from build123d import *

# Parameters (mm, degrees)
SKETCH1_W           = 76.2
SKETCH1_H           = 127
BOSS_EXTRUDE1_DEPTH = 2.54
SKETCH2_W           = 2.54
SKETCH2_H           = 25.4
CUT_EXTRUDE1_DEPTH  = 3.54
SKETCH4_W           = 2.54
SKETCH4_H           = 25.4
CUT_EXTRUDE3_DEPTH  = 3.54
SKETCH3_W           = 2.54
SKETCH3_H           = 25.4
CUT_EXTRUDE4_DEPTH  = 3.54


with BuildPart() as part:
    # Sketch1 → Boss-Extrude1 (new body)
    with BuildSketch(Plane.XY):
        with Locations((38.1, 63.5)):
            Rectangle(SKETCH1_W, SKETCH1_H)
    extrude(amount=BOSS_EXTRUDE1_DEPTH)

    # Sketch2 → Cut-Extrude1 (cut, through all)
    with BuildSketch(Plane.XY.offset(2.54)):
        with Locations((1.27, 114.3)):
            Rectangle(SKETCH2_W, SKETCH2_H)
    extrude(amount=-CUT_EXTRUDE1_DEPTH, mode=Mode.SUBTRACT)

    # Sketch4 → Cut-Extrude3 (cut, through all)
    with BuildSketch(Plane.XY.offset(2.54)):
        with Locations((1.27, 12.7)):
            Rectangle(SKETCH4_W, SKETCH4_H)
        with Locations((74.93, 12.7)):
            Rectangle(SKETCH4_W, SKETCH4_H)
        with Locations((1.27, 63.5)):
            Rectangle(SKETCH4_W, SKETCH4_H)
        with Locations((74.93, 63.5)):
            Rectangle(SKETCH4_W, SKETCH4_H)
    extrude(amount=-CUT_EXTRUDE3_DEPTH, mode=Mode.SUBTRACT)

    # Sketch3 → Cut-Extrude4 (cut, through all)
    with BuildSketch(Plane.XY.offset(2.54)):
        with Locations((74.93, 114.3)):
            Rectangle(SKETCH3_W, SKETCH3_H)
    extrude(amount=-CUT_EXTRUDE4_DEPTH, mode=Mode.SUBTRACT)


solid = part.part
Design review of the part built by this model. Coordinates are the model's own, in mm. A direction names the side the tool comes from. Coordinates: 2 decimals unless noted, no trailing zeros. Order: outer loops, then holes, each group sorted by start corner. A loop starts at its lowest first (then second) coordinate and runs counter-clockwise, first axis right, second up. Notation, with made-up numbers: (61, 60) -> (100, 60) arc R15 cw to (100, 66) -> close; hole circle Ø3 at (25.25, 55). An arc over 180 degrees is marked (long way). Use one line per item in the form item = value. Start each with the question number.
(1) Add section B-B on y = 10. State the section outline as (x, z) points, plus the area to 3 significant figures.
(2) For probe 1 along X at (y, z) = (7, 1.45), list the stretches that pass through material, from the lowest coordinate up.
(3) The part is to be moulded in two halves that separate along Y. For faces 1 (the flat face through (73.66, 63, 1)), 2 (the flat face through (2.54, 13, 1)), 3 (the flat face through (1, 25.4, 1)), say which applies: +Y half, -Y half, draft (parallel to the pull), parting line (faces both ways), or undercut.
(4) Insertion check: pin 1 (1.3 mm diameter, centred on y = 110, z = 1.5, fed in from -X); pin 2 (0.8 mm diameter, centred on x = 75, z = 1, fed in from -Y); pin 3 (0.8 mm diameter, centred on y = 118.5, z = 2, fed in from +X). Each pin has a flat end and moves straight along its axis. Give the tip position at first contact, or say it passes through.
(5) For faces 4 (the flat face through (2.54, 114, 1)), 5 (the flat face through (75, 25.4, 1)), 6 (the flat face through (73.66, 114, 1)), list the 3-axis set-ups (+Z, -Z, +X, -X, +Y, -Y) from which the entire face can be reached by the end or side of a thin tool; tool diameter is ignored.
(6) Add section A-A on z = 0.9. State the section outline as (x, y) points.
Answer block:
q1.outline = (2.54, 0) -> (73.66, 0) -> (73.66, 2.54) -> (2.54, 2.54) -> close
q1.area = 181 mm²
q2.probe_1 = 2.54 to 73.66
q3.face_1 = undercut
q3.face_2 = draft
q3.face_3 = -Y half
q4.pin_1 = 2.54
q4.pin_2 = 25.4
q4.pin_3 = 73.66
q5.face_4 = +Z, -Z, -X, +Y
q5.face_5 = +Z, -Z, +X, -Y
q5.face_6 = +Z, -Z, +X, +Y
q6.outline = (0, 25.4) -> (2.54, 25.4) -> (2.54, 0) -> (73.66, 0) -> (73.66, 25.4) -> (76.2, 25.4) -> (76.2, 50.8) -> (73.66, 50.8) -> (73.66, 76.2) -> (76.2, 76.2) -> (76.2, 101.6) -> (73.66, 101.6) -> (73.66, 127) -> (2.54, 127) -> (2.54, 101.6) -> (0, 101.6) -> (0, 76.2) -> (2.54, 76.2) -> (2.54, 50.8) -> (0, 50.8) -> close
